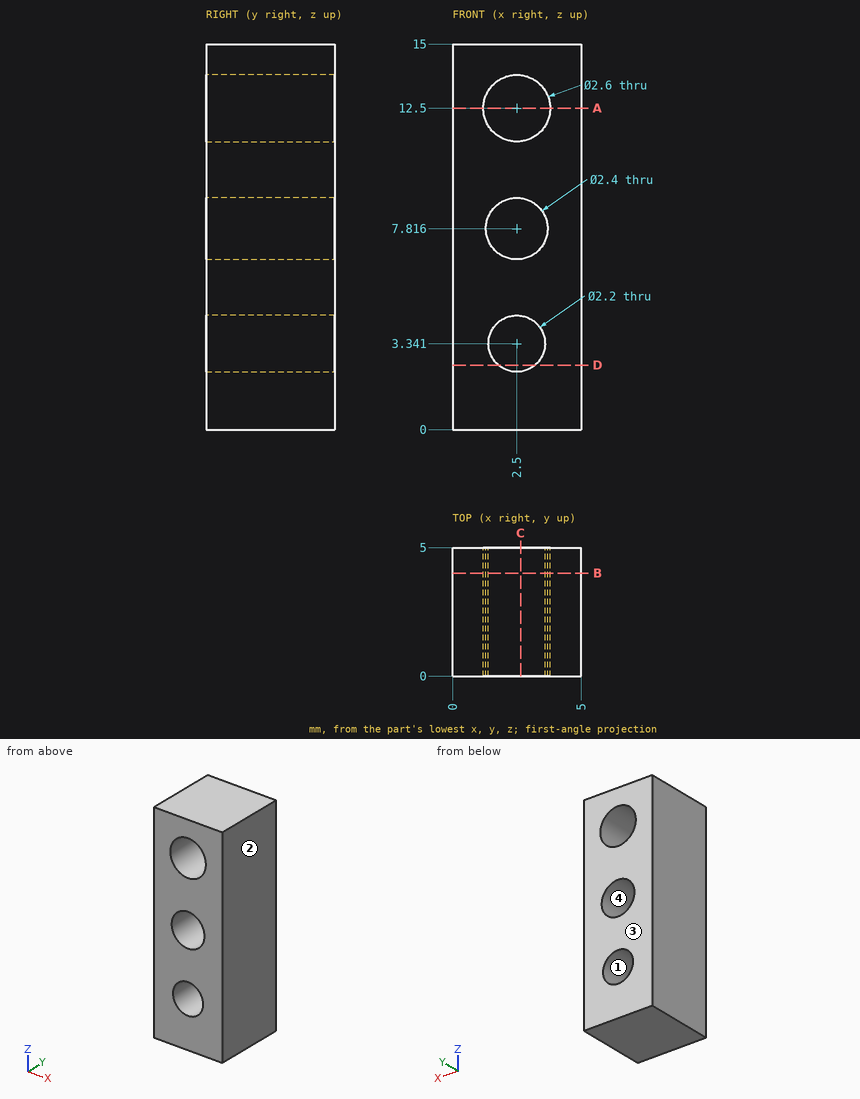
Part print with two shaded views. Sizes in mm from the minimum x, y, z corner. Round coordinates to 2 decimals unless told otherwise and drop trailing zeros. Order: outer loops, then holes, each group sorted by start corner. A loop starts at its lowest first (then second) coordinate and runs counter-clockwise, first axis right, second up. Notation, with made-up numbers: M 1.25,-6 L 46.25,-6 A25 cw 46.25,24 Z; hole C -0.75,-38.75 d9. An arc over 180 degrees is marked long. Answer in a Markdown table with one row per item. Add a question column.
Q1. Cut at B-B on y = 4. Give the cut face in (x, z) (1 decimal).
Q2. Cut at D-D on z = 2.5. Give the cut face in (x, y).
Q3. Mould opens along X. For the marked faces 1, 2, 3 and 4 say: +X half, -X half, draft (parallel to the pull), parting line (faces both ways), or undercut.
Q4. Cut at C-C on x = 2.65. Give the cut face in (y, z) (1 decimal).
Q5. Wall check: L1, parallel to Z at x = 3, y = 0.95 (1 decimal); L2, parallel to Z at x = 1.8, y = 1.7 (1 decimal); L3, parallel to X at y = 1.1, z = 12.5. Give the ranges that are in metal, low to high. Write a range as from..to.
Q6. Pin check, flat tips, straight feed: pin 1 (3 mm diameter, centred on x = 2.5, z = 7.82, fed in from +Y); pin 2 (1.8 mm diameter, centred on x = 2.5, z = 3.34, fed in from +Y). Stop position of each tip, or through.
Q7. Cut at A-A on z = 12.5. Give the cut face in (x, y).
Established:
| question | item | result |
|---|---|---|
| 1 | outline | M 0,0 L 5,0 L 5,15 L 0,15 Z; hole C 2.5,12.5 d2.6; hole C 2.5,7.8 d2.4; hole C 2.5,3.3 d2.2 |
| 2 | outline | M 0,0 L 1.79,0 L 1.79,5 L 0,5 Z; M 3.21,0 L 5,0 L 5,5 L 3.21,5 Z |
| 3 | face 1 | undercut |
| 3 | face 2 | +X half |
| 3 | face 3 | draft |
| 3 | face 4 | undercut |
| 4 | outline | M 0,0 L 5,0 L 5,2.3 L 0,2.3 Z; M 0,4.4 L 5,4.4 L 5,6.6 L 0,6.6 Z; M 0,9 L 5,9 L 5,11.2 L 0,11.2 Z; M 0,13.8 L 5,13.8 L 5,15 L 0,15 Z |
| 5 | L1 | z = 0..2.4, 4.3..6.7, 8.9..11.3, 13.7..15 |
| 5 | L2 | z = 0..2.5, 4.2..6.8, 8.8..11.4, 13.6..15 |
| 5 | L3 | x = 0..1.2, 3.8..5 |
| 6 | pin 1 | stops at y = 5 |
| 6 | pin 2 | passes through |
| 7 | outline | M 0,0 L 1.2,0 L 1.2,5 L 0,5 Z; M 3.8,0 L 5,0 L 5,5 L 3.8,5 Z |
